```python
from build123d import *

# Parameters (mm, degrees)
SKETCH1_R           = 6.35
BOSS_EXTRUDE1_DEPTH = 6.35
SKETCH2_R           = 4.7625
BOSS_EXTRUDE2_DEPTH = 7.9375
SKETCH3_R           = 3.175
CUT_EXTRUDE1_DEPTH  = 14.2875


with BuildPart() as part:
    # Sketch1 → Boss-Extrude1 (new body)
    with BuildSketch(Plane.XY):
        Circle(SKETCH1_R)
    extrude(amount=BOSS_EXTRUDE1_DEPTH)

    # Sketch2 → Boss-Extrude2 (add)
    with BuildSketch(Plane(origin=(0, 0, 0), x_dir=(-1, 0, 0), z_dir=(0, 0, -1))):
        with Locations(Location((0, 0, 0), (0, 0, 180))):
            Circle(SKETCH2_R)
    extrude(amount=BOSS_EXTRUDE2_DEPTH)

    # Sketch3 → Cut-Extrude1 (cut)
    with BuildSketch(Plane(origin=(0, 0, -7.9375), x_dir=(-1, 0, 0), z_dir=(0, 0, -1))):
        Circle(SKETCH3_R)
    extrude(amount=-CUT_EXTRUDE1_DEPTH, mode=Mode.SUBTRACT)


solid = part.part
```
The listing builds one solid part. Answer for the finished solid, in the listing's coordinates (mm). A direction names the side the tool comes from. Round coordinates to 2 decimals unless told otherwise and drop trailing zeros. Loops run counter-clockwise (first coordinate to the right, second up) from the corner with the lowest first, then second, coordinate; pieces in that order, holes last.
1) For faces 1 (the face through (1, 5, 0)), 2 (the face through (-1.38, -6.2, 3.13)), determine the directions among +Z, -Z, +X, -X, +Y, -Y from which every point of the face is accessible in a straight line to the end or side of a thin tool.
Outcome:
face 1: -Z
face 2: +Z, -Z
2) A cutting plane is placed at D-D on y = 5.75. Determine the outline of the cut face in (x, z).
Outcome:
outline: (-2.69, 0) - (2.69, 0) - (2.69, 6.35) - (-2.69, 6.35) - close
3) Consider line 1 (Y direction, x = 0, z = 2.25) (3 decimals); line 2 (Y direction, x = 0, z = -3.25) (1 decimal); line 3 (Z direction, x = 5.5, y = 1). Determine where each line is inside the solid, lowest interval first.
Outcome:
line 1: y = -6.35 to -3.175, 3.175 to 6.35
line 2: y = -4.8 to -3.2, 3.2 to 4.8
line 3: z = 0 to 6.35
4) Given P1, Ø1, axis at y = 2.5, z = 1, coming from the -X side; P2, Ø6, axis at y = -4.5, z = -2.5, coming from the -X side, each flat-ended and moving along its own axis, determine where each tip first touches the part or whether it passes through.
Outcome:
P1: stops at x = -6.03
P2: stops at x = -5.68
